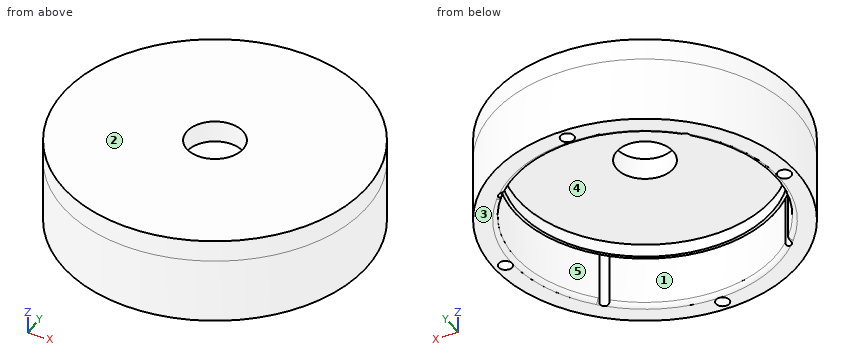
```python
from build123d import *

# Parameters (mm, degrees)
SKETCH_2_R          = 35
SKETCH_2_R_2        = 6.5
EXTRUDE_1_DEPTH     = 5
EXTRUDE_START       = 15
SKETCH_3_R          = 35
SKETCH_3_R_2        = 30
EXTRUDE_2_DEPTH     = 15
SKETCH_4_R          = 1.55
CUT_EXTRUDE_1_DEPTH = 10
CUT_EXTRUDE_5_DEPTH = 15
FILLET_1_R          = 1
EXTRUDE_START_2     = 3
SKETCH_10_R         = 30
SKETCH_10_R_2       = 29.3
EXTRUDE_3_DEPTH     = 3


with BuildPart() as part:
    # 草图2 → 凸台-拉伸1 (new body)
    with BuildSketch(Plane.XY):
        Circle(SKETCH_2_R)
        Circle(SKETCH_2_R_2, mode=Mode.SUBTRACT)
    extrude(amount=EXTRUDE_1_DEPTH)

    # 草图3 → 凸台-拉伸2 (add)
    with BuildSketch(Plane(origin=(0, 0, 0), x_dir=(-1, 0, 0), z_dir=(0, 0, -1)).offset(EXTRUDE_START)):
        Circle(SKETCH_3_R)
        Circle(SKETCH_3_R_2, mode=Mode.SUBTRACT)
    extrude(amount=-EXTRUDE_2_DEPTH)

    # 草图4 → 切除-拉伸1 (cut)
    with BuildSketch(Plane(origin=(0, 0, -15), x_dir=(-1, 0, 0), z_dir=(0, 0, -1))):
        with Locations((0, 32.5)):
            Circle(SKETCH_4_R)
        with Locations((32.5, 0)):
            Circle(SKETCH_4_R)
        with Locations((0, -32.5)):
            Circle(SKETCH_4_R)
        with Locations((-32.5, 0)):
            Circle(SKETCH_4_R)
    extrude(amount=-CUT_EXTRUDE_1_DEPTH, mode=Mode.SUBTRACT)

    # 草图9 → 切除-拉伸5 (cut)
    with BuildSketch(Plane(origin=(0, 0, -15), x_dir=(-1, 0, 0), z_dir=(0, 0, -1))):
        with BuildLine():
            ThreePointArc((-21.942558771, 20.457861926), (-21.955665556, 21.955665556), (-20.457861926, 21.942558771))
            ThreePointArc((-20.457861926, 21.942558771), (-21.213203436, 21.213203436), (-21.942558771, 20.457861926))
        make_face()
        with BuildLine():
            ThreePointArc((20.457861926, 21.942558771), (21.955665556, 21.955665556), (21.942558771, 20.457861926))
            ThreePointArc((21.942558771, 20.457861926), (21.213203436, 21.213203436), (20.457861926, 21.942558771))
        make_face()
        with BuildLine():
            ThreePointArc((21.942558771, -20.457861926), (21.955665556, -21.955665556), (20.457861926, -21.942558771))
            ThreePointArc((20.457861926, -21.942558771), (21.213203436, -21.213203436), (21.942558771, -20.457861926))
        make_face()
        with BuildLine():
            ThreePointArc((-20.457861926, -21.942558771), (-21.955665556, -21.955665556), (-21.942558771, -20.457861926))
            ThreePointArc((-21.942558771, -20.457861926), (-21.213203436, -21.213203436), (-20.457861926, -21.942558771))
        make_face()
    extrude(amount=-CUT_EXTRUDE_5_DEPTH, mode=Mode.SUBTRACT)

    # 圆角1
    # the kernel refuses this fillet: 1 mm, written as the material it takes off along each edge
    with BuildSketch(Plane(origin=(0, 0, -15), x_dir=(-0.740463861633537, 0.6720961758667804, 0), z_dir=(-0.6720961758667804, -0.740463861633537, 0))) as fillet_1_piece_1:
        with BuildLine():
            CenterArc((30 + FILLET_1_R, -FILLET_1_R), FILLET_1_R, 90, 90)
            Line((30, -FILLET_1_R), (30, 0))
            Line((30, 0), (30 + FILLET_1_R, 0))
        make_face()
    revolve(axis=Axis((0, 0, -15), (0, 0, -1)), revolution_arc=95.541888931, mode=Mode.SUBTRACT)
    with BuildSketch(Plane(origin=(0, 0, -15), x_dir=(0.6720961758667806, 0.7404638616335367, 0), z_dir=(-0.7404638616335367, 0.6720961758667806, 0))) as fillet_1_piece_2:
        with BuildLine():
            CenterArc((30 + FILLET_1_R, -FILLET_1_R), FILLET_1_R, 90, 90)
            Line((30, -FILLET_1_R), (30, 0))
            Line((30, 0), (30 + FILLET_1_R, 0))
        make_face()
    revolve(axis=Axis((0, 0, -15), (0, 0, -1)), revolution_arc=95.541888931, mode=Mode.SUBTRACT)
    with BuildSketch(Plane(origin=(0, 0, -15), x_dir=(0.7404638616335368, -0.6720961758667805, 0), z_dir=(0.6720961758667805, 0.7404638616335368, 0))) as fillet_1_piece_3:
        with BuildLine():
            CenterArc((30 + FILLET_1_R, -FILLET_1_R), FILLET_1_R, 90, 90)
            Line((30, -FILLET_1_R), (30, 0))
            Line((30, 0), (30 + FILLET_1_R, 0))
        make_face()
    revolve(axis=Axis((0, 0, -15), (0, 0, -1)), revolution_arc=95.541888931, mode=Mode.SUBTRACT)
    with BuildSketch(Plane(origin=(0, 0, -15), x_dir=(-1, 0, 0), z_dir=(0, -1, 0))) as fillet_1_piece_4:
        with BuildLine():
            CenterArc((30 + FILLET_1_R, -FILLET_1_R), FILLET_1_R, 90, 90)
            Line((30, -FILLET_1_R), (30, 0))
            Line((30, 0), (30 + FILLET_1_R, 0))
        make_face()
    revolve(axis=Axis((0, 0, -15), (0, 0, -1)), revolution_arc=47.769631262, mode=Mode.SUBTRACT)
    with BuildSketch(Plane(origin=(0, 0, -15), x_dir=(-0.6721131469252694, -0.7404484571732264, 0), z_dir=(0.7404484571732264, -0.6721131469252694, 0))) as fillet_1_piece_5:
        with BuildLine():
            CenterArc((30 + FILLET_1_R, -FILLET_1_R), FILLET_1_R, 90, 90)
            Line((30, -FILLET_1_R), (30, 0))
            Line((30, 0), (30 + FILLET_1_R, 0))
        make_face()
    revolve(axis=Axis((0, 0, -15), (0, 0, -1)), revolution_arc=47.769631262, mode=Mode.SUBTRACT)

    # 草图10 → 凸台-拉伸3 (add)
    with BuildSketch(Plane(origin=(0, 0, 0), x_dir=(-1, 0, 0), z_dir=(0, 0, -1)).offset(EXTRUDE_START_2)):
        Circle(SKETCH_10_R)
        Circle(SKETCH_10_R_2, mode=Mode.SUBTRACT)
    extrude(amount=-EXTRUDE_3_DEPTH)


solid = part.part
```
For this review, take the finished solid that the model builds, in its own axes (mm). Face numbers are marked on the shaded views. A direction names the side the tool comes from. Coordinates: 2 decimals unless noted, no trailing zeros. Loops run counter-clockwise (first coordinate to the right, second up) from the corner with the lowest first, then second, coordinate; pieces in that order, holes last. Notation, with made-up numbers: (71, -37) -> (127, -37) arc R28 cw to (127, -5) -> close; hole circle Ø1 at (20.25, -40). An arc over 180 degrees is marked (long way). Return JSON: item names as keys, results as strings. Group by question number.
(1) Mouldability with a two-part tool opening along X and no side actions: class the marked faces 3, 4 and 5 as pulls with the +X half, pulls with the -X half, needs draft (parallel to the pull), parting line crosses it, or undercut.
(2) Consider section B-B, the plane x = 32.5. Give the boundary of the cut face in (y, z).
(3) For pin 1 Ø1 at (x, z) = (-21.5, -12) entering from -Y; pin 2 Ø18 at (x, y) = (-8, 6.5) entering from -Z; pin 3 Ø1 at (x, z) = (3.5, -5.5) entering from +Y, all flat-tipped, find the tip position at first contact; note any pin that passes through.
(4) Consider section A-A, the plane z = -10.5. Give the boundary of the cut face in (x, y).
(5) Tool access review of the marked faces 1 and 2: name each direction out of +Z, -Z, +X, -X, +Y, -Y from which nothing blocks a thin tool from reaching the whole face with its end or side.
(6) Consider section D-D, the plane z = 1.5. Give the boundary of the cut face in (x, y).
(7) To check wall thickness, follow L1, parallel to X at y = 0, z = -11.25; L2, parallel to Y at x = 0, z = 3.4; L3, parallel to Y at x = 0, z = -1.55. State the ranges of each line that lie inside material, in increasing order.
Results below:
{
 "1": {"face 3": "needs draft", "face 4": "undercut", "face 5": "undercut"},
 "2": {"outline": "(-12.99, -15) -> (-1.55, -15) -> (-1.55, -5) -> (1.55, -5) -> (1.55, -15) -> (12.99, -15) -> (12.99, 5) -> (-12.99, 5) -> close"},
 "3": {"pin 1": "stops at y = -28", "pin 2": "stops at z = 0", "pin 3": "stops at y = 34.87"},
 "4": {"outline": "circle Ø70 at (0, 0); hole circle Ø3.1 at (-32.5, 0); hole (-21.94, -20.46) arc R1.05 ccw (long way) to (-20.46, -21.94) arc R30 ccw to (20.46, -21.94) arc R1.05 ccw (long way) to (21.94, -20.46) arc R30 ccw to (21.94, 20.46) arc R1.05 ccw (long way) to (20.46, 21.94) arc R30 ccw to (-20.46, 21.94) arc R1.05 ccw (long way) to (-21.94, 20.46) arc R30 ccw to start; hole circle Ø3.1 at (0, -32.5); hole circle Ø3.1 at (0, 32.5); hole circle Ø3.1 at (32.5, 0)"},
 "5": {"face 1": "-Z", "face 2": "+Z, +X, -X, +Y, -Y"},
 "6": {"outline": "circle Ø70 at (0, 0); hole circle Ø13 at (0, 0)"},
 "7": {"L1": "x = -35 to -34.05, -30.95 to -30, 30 to 30.95, 34.05 to 35", "L2": "y = -35 to -6.5, 6.5 to 35", "L3": "y = -35 to -29.3, 29.3 to 35"}
}
